Check sheet for the modelled part. Datum: model origin and axes. Units: mm. A direction names the side the tool comes from. Give positions to 0.01 mm unless a question says otherwise; leave off trailing zeros. Loops run counter-clockwise (first coordinate to the right, second up) from the corner with the lowest first, then second, coordinate; pieces in that order, holes last. Notation, with made-up numbers: M 46.25,62 L 60.25,62 A31 ccw 60.25,97 Z; hole C 47,62 d8. An arc over 180 degrees is marked long. Use one line per item in the form item = value.
from build123d import *

# Parameters (mm, degrees)
SKETCH_1_R          = 22.5
SKETCH_1_R_2        = 1.55
EXTRUDE_1_DEPTH     = 2
SKETCH_2_R          = 4.98
EXTRUDE_2_DEPTH     = 3
SKETCH_3_R          = 6
EXTRUDE_3_DEPTH     = 0.5
SKETCH_4_R          = 3
CUT_EXTRUDE_1_DEPTH = 33.210246817


with BuildPart() as part:
    # ｽｹｯﾁ1 → ﾎﾞｽ - 押し出し1 (new body)
    with BuildSketch(Plane(origin=(0, 0, 0), x_dir=(1, 0, 0), z_dir=(0, 1, 0))):
        with Locations(Location((0, 0, 0), (0, 0, 270))):
            Circle(SKETCH_1_R)
        with Locations(Location((0, 16, 0), (0, 0, 270))):
            Circle(SKETCH_1_R_2, mode=Mode.SUBTRACT)
        with Locations(Location((13.856406461, -8, 0), (0, 0, 270))):
            Circle(SKETCH_1_R_2, mode=Mode.SUBTRACT)
        with Locations(Location((-13.856406461, -8, 0), (0, 0, 270))):
            Circle(SKETCH_1_R_2, mode=Mode.SUBTRACT)
    extrude(amount=EXTRUDE_1_DEPTH)

    # ｽｹｯﾁ2 → ﾎﾞｽ - 押し出し2 (add)
    with BuildSketch(Plane(origin=(0, 2, 0), x_dir=(1, 0, 0), z_dir=(0, 1, 0))):
        with Locations(Location((0, 0, 0), (0, 0, 270))):
            Circle(SKETCH_2_R)
    extrude(amount=EXTRUDE_2_DEPTH)

    # ｽｹｯﾁ3 → ﾎﾞｽ - 押し出し3 (add)
    with BuildSketch(Plane(origin=(0, 2, 0), x_dir=(1, 0, 0), z_dir=(0, 1, 0))):
        with Locations(Location((0, 0, 0), (0, 0, 270))):
            Circle(SKETCH_3_R)
    extrude(amount=EXTRUDE_3_DEPTH)

    # ｽｹｯﾁ4 → ｶｯﾄ - 押し出し1 (cut, through all)
    with BuildSketch(Plane(origin=(0, 5, 0), x_dir=(1, 0, 0), z_dir=(0, 1, 0))):
        with Locations(Location((0, 0, 0), (0, 0, 270))):
            Circle(SKETCH_4_R)
    extrude(amount=-CUT_EXTRUDE_1_DEPTH, mode=Mode.SUBTRACT)


solid = part.part
1) Depth check by flat-ended pin: pin 1 Ø3.5 at (x, z) = (0, -16) entering from +Y; pin 2 Ø1 at (y, z) = (2, 5.5) entering from -X. Enter the tip coordinate at first touch or a pass-through.
Evaluation:
pin_1 = 2
pin_2 = -21.94
2) Release check for a two-part mould opening along Z. For faces 1 (the face through (-3.3, 5, -0.1)), 2 (the face through (0.9, 2.54, 2.86)), 3 (the face through (1.802, 2.246, 5.723)), 4 (the face through (-12.549, 0.986, 8.833)) record: pulls with the +Z half, pulls with the -Z half, needs draft (parallel to the pull), parting line crosses it, or undercut.
Evaluation:
face_1 = needs draft
face_2 = undercut
face_3 = parting line crosses it
face_4 = undercut
3) Set-up check for faces 5 (the face through (-8.618, 0.986, 20.784)), 6 (the face through (-5, 2, 5)): record each of +Z, -Z, +X, -X, +Y, -Y from which the full face is reachable in a straight line by a thin tool's end or side.
Evaluation:
face_5 = +Y, -Y
face_6 = +Y
4) Section check B-B (z = 0). Record the cut outline in (x, y), then the cut area to 3 significant figures.
Evaluation:
outline = M -22.5,0 L -3,0 L -3,5 L -4.98,5 L -4.98,2.5 L -6,2.5 L -6,2 L -22.5,2 Z; M 3,0 L 22.5,0 L 22.5,2 L 6,2 L 6,2.5 L 4.98,2.5 L 4.98,5 L 3,5 Z
area = 90.9 mm^2
5) Section check A-A (x = 0). Record the cut outline in (y, z), then the cut area to 3 significant figures.
Evaluation:
outline = M 0,-22.5 L 2,-22.5 L 2,-17.55 L 0,-17.55 Z; M 0,-14.45 L 2,-14.45 L 2,-6 L 2.5,-6 L 2.5,-4.98 L 5,-4.98 L 5,-3 L 0,-3 Z; M 0,3 L 5,3 L 5,4.98 L 2.5,4.98 L 2.5,6 L 2,6 L 2,22.5 L 0,22.5 Z
area = 84.7 mm^2
6) Section check C-C (z = 9). Record the cut outline in (x, y).
Evaluation:
outline = M -20.62,0 L -15.04,0 L -15.04,2 L -20.62,2 Z; M -12.67,0 L 12.67,0 L 12.67,2 L -12.67,2 Z; M 15.04,0 L 20.62,0 L 20.62,2 L 15.04,2 Z
7) Section check D-D (y = 3.8). Record the cut outline in (x, z), then the cut area to 3 significant figures.
Evaluation:
outline = C 0,0 d9.96; hole C 0,0 d6
area = 49.6 mm^2
8) Scan lines: line 1 (X direction, y = 2.25, z = 0); line 2 (Y direction, x = -9, z = 1); line 3 (X direction, y = 0.9, z = 7). Record each from-to range of solid material in increasing order.
Evaluation:
line_1 = -6 to -3, 3 to 6
line_2 = 0 to 2
line_3 = -21.38 to -15.04, -12.67 to 12.67, 15.04 to 21.38
